from build123d import *

# Parameters (mm, degrees)
F1_DEPTH = 80
F2_W     = 50
F2_H     = 80
F2_R     = 15
F3_DEPTH = 15


with BuildPart() as f1:
    # F0 (on Front) → F1 (new body)
    with BuildSketch(Plane.XZ):
        Polygon((7.260843, 50), (-42.739157, 50), (-42.739157, -50), (22.260843, -50), (22.260843, -31.529605), (42.260843, -31.529605), (42.260843, -50), (57.260843, -50), (57.260843, 0), (7.260843, 0), align=None)
    extrude(amount=F1_DEPTH)

    # F2 (on face) → F3 (join)
    with BuildSketch(Plane.XY.offset(50)):
        with Locations((-17.739157, -40)):
            Rectangle(F2_W, F2_H)
        with Locations((-17.739157, -40)):
            Circle(F2_R, mode=Mode.SUBTRACT)
    extrude(amount=F3_DEPTH)


solid = f1.part
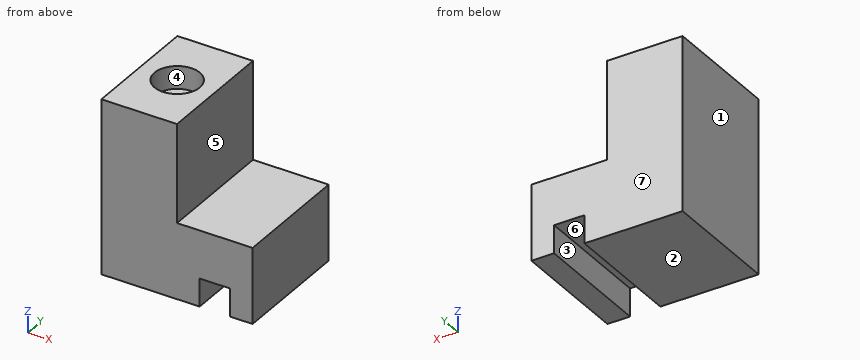
Geometry: final body of the model. Coordinates: model frame, mm. Face numbers are marked on the shaded views. A direction names the side the tool comes from. Give positions to 0.01 mm unless a question says otherwise; leave off trailing zeros. Write each loop counter-clockwise with the first axis right and the second up, starting at its lowest first coordinate (ties: lowest second). Pieces come first, ordered by that corner, then holes. Notation, with made-up numbers: (-16, 11.25) - (8, 11.25) arc R25 ccw to (8, 41.25) - close; hole circle Ø1 at (-28, -30.5). An arc over 180 degrees is marked (long way). Return JSON: item names as keys, results as strings. Group by question number.
1) Set-up query: the marked faces 4, 5, 6 and 7. Return all of +Z, -Z, +X, -X, +Y, -Y with unobstructed straight access to the full face (end or side cutting, diameter ignored); none if empty.
2) Line query: line 1 (X direction, y = -25, z = 25.5); line 2 (Z direction, x = 43.5, y = -23.5); line 3 (X direction, y = -20, z = -44). Output: solid intervals per line, ascending.
3) Section A-A on y = -40. Return the cut outline in (x, z), plus the area to 3 significant figures.
4) Mould query, pull axis X, two halves, no side actions, for the marked faces 1, 2 and 3. Classes: released by +X, released by -X, zero draft, split by the parting line, or undercut.
5) Section C-C on z = 29. Return the cut outline in (x, y).
6) First-contact query: P1, Ø3, axis at y = -45, z = 5.5, coming from the +X side; P2, Ø1.5, axis at x = 43, y = -59, coming from the +Z side; P3, Ø15, axis at x = -20, y = -41, coming from the +Z side; P4, Ø16, axis at x = 29.5, y = -59.5, coming from the -Z side. Flat tips, straight axial feed; report the tip coordinate or a pass-through.
7) Section B-B on x = -17. Return the cut outline in (y, z), plus the area to 3 significant figures.
8) Section D-D on y = -61. Return the cut outline in (x, z), plus the area to 3 significant figures.
Filled in:
{
 "1": {"face 4": "+Z", "face 5": "+Z, +X, +Y, -Y", "face 6": "-Z, +Y, -Y", "face 7": "+Z, -Z, +X, -X, +Y"},
 "2": {"line 1": "x = -42.74 to 7.26", "line 2": "z = -50 to 0", "line 3": "x = -42.74 to 22.26, 42.26 to 57.26"},
 "3": {"outline": "(-42.74, -50) - (22.26, -50) - (22.26, -31.53) - (42.26, -31.53) - (42.26, -50) - (57.26, -50) - (57.26, 0) - (7.26, 0) - (7.26, 65) - (-2.74, 65) - (-2.74, 50) - (-32.74, 50) - (-32.74, 65) - (-42.74, 65) - close", "area": "7,430 mm^2"},
 "4": {"face 1": "released by -X", "face 2": "zero draft", "face 3": "undercut"},
 "5": {"outline": "(-42.74, -80) - (7.26, -80) - (7.26, 0) - (-42.74, 0) - close"},
 "6": {"P1": "stops at x = 7.26", "P2": "stops at z = 0", "P3": "stops at z = 50", "P4": "stops at z = -50"},
 "7": {"outline": "(-80, -50) - (0, -50) - (0, 65) - (-25.02, 65) - (-25.02, 50) - (-54.98, 50) - (-54.98, 65) - (-80, 65) - close", "area": "8,750 mm^2"},
 "8": {"outline": "(-42.74, -50) - (22.26, -50) - (22.26, -31.53) - (42.26, -31.53) - (42.26, -50) - (57.26, -50) - (57.26, 0) - (7.26, 0) - (7.26, 65) - (-42.74, 65) - close", "area": "7,880 mm^2"}
}
